Model file for the job. Use its own axes, mm. Face numbers are marked on the shaded views. Give positions to 0.01 mm unless a question says otherwise; leave off trailing zeros. Write each loop counter-clockwise with the first axis right and the second up, starting at its lowest first coordinate (ties: lowest second). Pieces come first, ordered by that corner, then holes. Notation, with made-up numbers: (-8.75, -33.5) - (43.25, -33.5) arc R22 cw to (43.25, -5.5) - close; hole circle Ø2 at (89, 33.5). An arc over 180 degrees is marked (long way). One line per item, written item: value. Start each with the question number.
(1) Cut at A-A, the plane z = 4.5. List the corners of the cut face in (x, y) (1 decimal).
(2) Cut at B-B, the plane z = 0.75. List the corners of the cut face in (x, y) (1 decimal).
(3) Drop a flat-ended pin along its axis: P1, Ø4, axis at x = 4, y = -6.5, coming from the -Z side. Give the stop position or say it passes through.
(4) Mould opens along X. For the marked faces 1, 2, 3 and 4 say: pulls with the +X half, pulls with the -X half, needs draft (parallel to the pull), parting line crosses it, or undercut.
(5) Probe L1, parallel to Y at x = 0, z = 4.5; L2, parallel to Y at x = 9, z = 2.5; L3, parallel to X at y = -6.5, z = 5.25. List the from-to ranges inside material, lowest first.
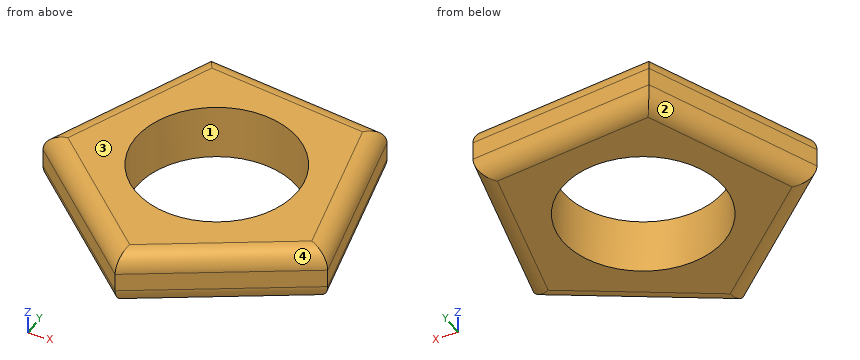
from build123d import *

# Parameters (mm, degrees)
F0_R     = 11.1125
F1_DEPTH = 7.62
F2_R     = 2.54


with BuildPart() as f1:
    # F0 (on Top) → F1 (new body)
    with BuildSketch(Plane.XY):
        Polygon((-2.56667, -21.73599), (19.87901, -9.157839), (14.852574, 16.076135), (-10.699615, 19.093436), (-21.4653, -4.275742), align=None)
        Circle(F0_R, mode=Mode.SUBTRACT)
    extrude(amount=F1_DEPTH)

    # F2
    f2_edges = [f1.edges().sort_by_distance(p)[0] for p in [
        (-12.015985, -13.005866, 7.62),
        (8.65617, -15.446914, 7.62),
        (17.365792, 3.459148, 7.62),
        (2.07648, 17.584785, 7.62),
        (-16.082457, 7.408847, 7.62),
        (8.65617, -15.446914, 0),
        (-12.015985, -13.005866, 0),
        (-16.082457, 7.408847, 0),
        (2.07648, 17.584785, 0),
        (17.365792, 3.459148, 0),
    ]]
    fillet(f2_edges, radius=F2_R)


solid = f1.part
Answers follow:
1. outline: (-21.5, -4.3) - (-2.6, -21.7) - (19.9, -9.2) - (14.9, 16.1) - (-10.7, 19.1) - close; hole circle Ø22.2 at (0, 0)
2. outline: (-20.6, -4.1) - (-2.5, -20.8) - (19.1, -8.8) - (14.2, 15.4) - (-10.3, 18.3) - close; hole circle Ø22.2 at (0, 0)
3. P1: passes through
4. face 1: undercut
4. face 2: pulls with the -X half
4. face 3: needs draft
4. face 4: pulls with the +X half
5. L1: y = -20.3 to -11.11, 11.11 to 17.83
5. L2: y = -15.25 to -6.52, 6.52 to 16.77
5. L3: x = -19.05 to -9.01, 9.01 to 19.34
